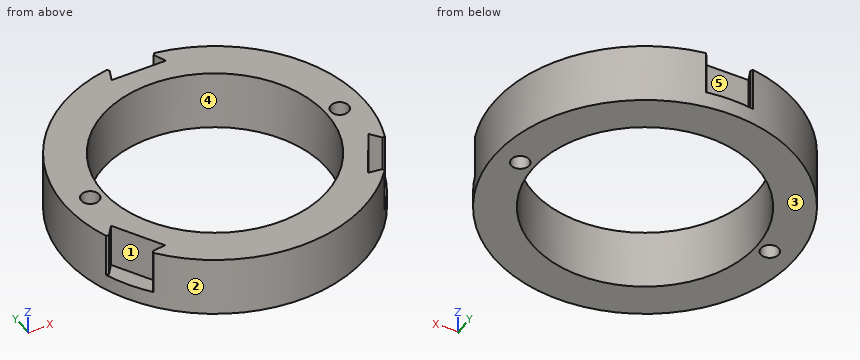
```python
from build123d import *

# Parameters (mm, degrees)
F0_R        = 27.5
F0_R_2      = 20.5
F1_DEPTH    = 11
F2_R        = 1.65
F3_DEPTH    = 11.001
F5_DEPTH    = 8
F6_T1_DEPTH = 9.2955577349


# Not quite as in the source:
# - a fillet or chamfer that OpenCascade refuses, or shapes differently, is made with other operations: its cross-section is extruded or revolved along the edge and cut away or added


with BuildPart() as f1:
    # F0 (on Top) → F1 (new body)
    with BuildSketch(Plane.XY):
        Circle(F0_R)
        Circle(F0_R_2, mode=Mode.SUBTRACT)
    extrude(amount=F1_DEPTH)

    # F2 (on face) → F3 (cut, through all)
    with BuildSketch(Plane.XY.offset(11)):
        with Locations((-23, 0)):
            Circle(F2_R)
        with Locations((23, 0)):
            Circle(F2_R)
    extrude(amount=-F3_DEPTH, mode=Mode.SUBTRACT)

    # F4 (on face) → F5 (cut)
    with BuildSketch(Plane.XY.offset(11)):
        Polygon((2.5, 30.5), (-2.5, 30.5), (-5, 24.5), (5, 24.5), align=None)
        Polygon((-27.6637748154, -13.0849364905), (-25.1637748154, -17.4150635095), (-18.7176223927, -16.5801270189), (-23.7176223927, -7.9198729811), align=None)
        Polygon((25.1637748154, -17.4150635095), (27.6637748154, -13.0849364905), (23.7176223927, -7.9198729811), (18.7176223927, -16.5801270189), align=None)
    extrude(amount=-F5_DEPTH, mode=Mode.SUBTRACT)

    # F6: chamfer of 0.5 on 6 edges, made by hand

    # F6_s2 → F6_t1 (cut)
    with BuildSketch(Plane.XY.offset(3)):
        with BuildLine():
            Line((4.3783542155, 27.1669165233), (4.0456541802, 26.7450037593))
            Line((4.0456541802, 26.7450037593), (4.0364234109, 26.7411576055))
            ThreePointArc((4.0364234109, 26.7411576055), (3.953486728, 26.9856318529), (3.8544223971, 27.223386247))
            Line((3.8544223971, 27.223386247), (3.8650581311, 27.2371332126))
            ThreePointArc((3.8650581311, 27.2371332126), (4.1213755716, 27.1995287348), (4.3799418411, 27.1767896913))
            Line((4.3799418411, 27.1767896913), (4.3783542155, 27.1669165233))
        make_face()
        with BuildLine():
            Line((-4.3783542155, 27.1669165233), (-4.0456541802, 26.7450037593))
            Line((-4.0456541802, 26.7450037593), (-4.0364234109, 26.7411576055))
            ThreePointArc((-4.0364234109, 26.7411576055), (-3.953486728, 26.9856318529), (-3.8544223971, 27.223386247))
            Line((-3.8544223971, 27.223386247), (-3.8650581311, 27.2371332126))
            ThreePointArc((-3.8650581311, 27.2371332126), (-4.1213755716, 27.1995287348), (-4.3799418411, 27.1767896913))
            Line((-4.3799418411, 27.1767896913), (-4.3783542155, 27.1669165233))
        make_face()
        with BuildLine():
            Line((25.7164169594, -9.7916922843), (25.18467977, -9.8688625847))
            Line((25.18467977, -9.8688625847), (25.1767335184, -9.8749335884))
            ThreePointArc((25.1767335184, -9.8749335884), (25.3469860858, -10.0689959865), (25.5033552655, -10.2736654107))
            Line((25.5033552655, -10.2736654107), (25.520578354, -10.2713280777))
            ThreePointArc((25.520578354, -10.2713280777), (25.6161706411, -10.0305484239), (25.7257611865, -9.7952539442))
            Line((25.7257611865, -9.7952539442), (25.7164169594, -9.7916922843))
        make_face()
        with BuildLine():
            Line((21.3380627439, -17.3752242391), (21.1390255898, -16.8761411746))
            Line((21.1390255898, -16.8761411746), (21.1403101075, -16.866224017))
            ThreePointArc((21.1403101075, -16.866224017), (21.3934993578, -16.9166358664), (21.6489328684, -16.9497208363))
            Line((21.6489328684, -16.9497208363), (21.6555202229, -16.965805135))
            ThreePointArc((21.6555202229, -16.965805135), (21.4947950695, -17.168980311), (21.3458193454, -17.3815357471))
            Line((21.3458193454, -17.3815357471), (21.3380627439, -17.3752242391))
        make_face()
        with BuildLine():
            Line((-25.7164169594, -9.7916922843), (-25.18467977, -9.8688625847))
            Line((-25.18467977, -9.8688625847), (-25.1767335184, -9.8749335884))
            ThreePointArc((-25.1767335184, -9.8749335884), (-25.3469860858, -10.0689959865), (-25.5033552655, -10.2736654107))
            Line((-25.5033552655, -10.2736654107), (-25.520578354, -10.2713280777))
            ThreePointArc((-25.520578354, -10.2713280777), (-25.6161706411, -10.0305484239), (-25.7257611865, -9.7952539442))
            Line((-25.7257611865, -9.7952539442), (-25.7164169594, -9.7916922843))
        make_face()
        with BuildLine():
            Line((-21.3380627439, -17.3752242391), (-21.1390255898, -16.8761411746))
            Line((-21.1390255898, -16.8761411746), (-21.1403101075, -16.866224017))
            ThreePointArc((-21.1403101075, -16.866224017), (-21.3934993578, -16.9166358664), (-21.6489328684, -16.9497208363))
            Line((-21.6489328684, -16.9497208363), (-21.6555202229, -16.965805135))
            ThreePointArc((-21.6555202229, -16.965805135), (-21.4947950695, -17.168980311), (-21.3458193454, -17.3815357471))
            Line((-21.3458193454, -17.3815357471), (-21.3380627439, -17.3752242391))
        make_face()
    extrude(amount=F6_T1_DEPTH, mode=Mode.SUBTRACT)


solid = f1.part
```
Verification items for the finished model (mm, model axes). Face numbers are marked on the shaded views. A direction names the side the tool comes from. Round coordinates to 2 decimals unless told otherwise and drop trailing zeros. Write each loop counter-clockwise with the first axis right and the second up, starting at its lowest first coordinate (ties: lowest second). Pieces come first, ordered by that corner, then holes. Notation, with made-up numbers: (-9, -30) -> (14, -30) arc R8 ccw to (14, -19) -> close; hole circle Ø8 at (19.5, -33). An arc over 180 degrees is marked (long way). Write each question's results on one line, items separated by ' | '. Start each with the question number.
1. Cross-section at D-D (x = 0). Enter the section's corners in (y, z).
2. Set-up check for the marked faces 4 and 5: record each of +Z, -Z, +X, -X, +Y, -Y from which the full face is reachable in a straight line by a thin tool's end or side.
3. Cross-section at B-B (x = -16.5). Enter the section's corners in (y, z).
4. Cross-section at A-A (y = 0). Enter the section's corners in (x, z), then the cut area to 3 significant figures.
5. Material ranges on probe 1 along Y at (x, z) = (4.5, 9.25); probe 2 along Y at (x, z) = (-11, 8.25); probe 3 along X at (y, z) = (-10.5, 4.5), recorded low to high. Write a range as from..to.
6. Draft check along Y on the marked faces 1, 2 and 3. Enter one of: +Y half, -Y half, draft (parallel to the pull), parting line (faces both ways), or undercut.
7. Depth check by flat-ended pin: P1, Ø2, axis at y = -15.5, z = 6.5, coming from the -X side; P2, Ø4, axis at y = -10.5, z = 3.5, coming from the +X side; P3, Ø3, axis at x = -23, y = 0, coming from the +Z side; P4, Ø3.5, axis at x = -23.5, y = -12, coming from the +Z side. Enter the tip coordinate at first touch or a pass-through.
8. Cross-section at C-C (y = -12.5). Enter the section's corners in (x, z).
Solutions:
1) outline: (-27.5, 0) -> (-20.5, 0) -> (-20.5, 11) -> (-27.5, 11) -> close; (20.5, 0) -> (27.5, 0) -> (27.5, 3) -> (24.5, 3) -> (24.5, 11) -> (20.5, 11) -> close
2) face 4: +Z, -Z | face 5: +Z
3) outline: (-22, 0) -> (-12.17, 0) -> (-12.17, 11) -> (-22, 11) -> close; (12.17, 0) -> (22, 0) -> (22, 11) -> (12.17, 11) -> close
4) outline: (-27.5, 0) -> (-24.65, 0) -> (-24.65, 11) -> (-27.5, 11) -> close; (-21.35, 0) -> (-20.5, 0) -> (-20.5, 11) -> (-21.35, 11) -> close; (20.5, 0) -> (21.35, 0) -> (21.35, 11) -> (20.5, 11) -> close; (24.65, 0) -> (27.5, 0) -> (27.5, 11) -> (24.65, 11) -> close | area: 81.4 mm2
5) probe 1: y = -27.13..-20, 20..24.5, 25.7..27.13 | probe 2: y = -25.2..-17.3, 17.3..25.2 | probe 3: x = -22.23..-17.61, 17.61..22.23
6) face 1: undercut | face 2: parting line | face 3: draft
7) P1: stops at x = -19.92 | P2: stops at x = 26.15 | P3: passes through | P4: stops at z = 3
8) outline: (-24.49, 0) -> (-16.25, 0) -> (-16.25, 11) -> (-21.07, 11) -> (-21.07, 3) -> (-24.49, 3) -> close; (16.25, 0) -> (24.49, 0) -> (24.49, 3) -> (21.07, 3) -> (21.07, 11) -> (16.25, 11) -> close
